Autodesk Inventor part; units mm, degrees
ref_plane "YZ Plane" through (0, 0, 0) normal (1, 0, 0) x (0, 1, 0)
ref_plane "XZ Plane" through (0, 0, 0) normal (0, 1, 0) x (-1, 0, 0)
ref_plane "XY Plane" through (0, 0, 0) normal (0, 0, 1) x (1, 0, 0)
sketch "Sketch1" plane through (0, 0, 0) normal (0, 1, 0) x (-1, 0, 0)
  circle A0 centre (0, 0) radius 1.5
  dimension "d0" = 3
extrude "Extrusion1" add sketch "Sketch1" along normal blind 10
sketch "Sketch2" plane through (0, 0, 0) normal (0, -1, 0) x (1, 0, 0)
  circle A0 centre (0, 0) radius 2.5
  dimension "d3" = 5
extrude "Extrusion2" add sketch "Sketch2" along normal blind 3
fillet "Fillet1" radius 2 1 edges at (-2.5, -3, 0)
sketch "Sketch3" plane through (0, -3, 0) normal (0, -1, 0) x (1, 0, 0)
  circle A0 centre (0, 0) radius 0.5
  line L0 (-1.8667, 0) -> (-0.4174, -0.2753)
  circle A1 centre (0, 0) radius 0.5
  line L1 (-1.8667, 0) -> (-0.5, 0)
  dimension "d9" = 0
extrude "Extrusion3" cut sketch "Sketch3" against normal blind 2 contours A0 L0 L1
mirror "Mirror1" about plane through (0, 0, 0) normal (0, 0, 1) of "Extrusion3"
pattern_circular "Circular Pattern1" count 4 over 360 about axis through (0, -1, 0) along (0, -1, 0) of "Extrusion3", "Mirror1"
sketch "Sketch4" plane through (0, -3, 0) normal (0, -1, 0) x (1, 0, 0)
  arc A0 (-0.4174, 0.2753) -> (-0.4174, -0.2753) centre (0, 0) ccw
  arc A1 (-0.4174, -0.2753) -> (-0.2753, -0.4174) centre (0, 0) ccw
  arc A2 (-0.2753, -0.4174) -> (0.2753, -0.4174) centre (0, 0) ccw
  arc A3 (0.2753, -0.4174) -> (0.4174, -0.2753) centre (0, 0) ccw
  arc A4 (0.4174, -0.2753) -> (0.4174, 0.2753) centre (0, 0) ccw
  arc A5 (0.4174, 0.2753) -> (0.2753, 0.4174) centre (0, 0) ccw
  arc A6 (0.2753, 0.4174) -> (-0.2753, 0.4174) centre (0, 0) ccw
  arc A7 (-0.2753, 0.4174) -> (-0.4174, 0.2753) centre (0, 0) ccw
extrude "Extrusion4" cut sketch "Sketch4" against normal up to surface (2 mm away)
The model under review builds one solid part; all positions refer to its coordinate system, in mm. A direction names the side the tool comes from. Round coordinates to 2 decimals unless told otherwise and drop trailing zeros. Loops run counter-clockwise (first coordinate to the right, second up) from the corner with the lowest first, then second, coordinate; pieces in that order, holes last.
Item 1: For faces 1 (the face through (0, 10, 0)), 2 (the face through (0, -1, 0)), list the 3-axis set-ups (+Z, -Z, +X, -X, +Y, -Y) from which the entire face can be reached by the end or side of a thin tool; tool diameter is ignored.
Determined:
face 1: +Z, -Z, +X, -X, +Y
face 2: -Y
Item 2: Take a section at A-A (y = 1.25). Write out the cut boundary in (x, z), then the cut area to 3 significant figures.
Determined:
outline: circle Ø3 at (0, 0)
area: 7.07 mm2
Item 3: Clearance check with flat-ended pins moving along their axes: pin 1 Ø1.5 at (x, z) = (1, 1.5) entering from -Y; pin 2 Ø1 at (x, z) = (-1.5, 1.5) entering from -Y; pin 3 Ø2 at (x, y) = (0.5, 3.5) entering from +Z. State where each tip first meets the part, or that it passes through.
Determined:
pin 1: stops at y = -2.92
pin 2: stops at y = -2.66
pin 3: stops at z = 1.5
Item 4: Mouldability with a two-part tool opening along Z and no side actions: class faces 3 (the face through (1.5, 4.93, -0.07)), 4 (the face through (-1.152, -2.014, -0.136)), 5 (the face through (1.13, -2.01, -0.14)), 6 (the face through (2, 0, 0)) as released by +Z, released by -Z, zero draft, split by the parting line, or undercut.
Determined:
face 3: split by the parting line
face 4: undercut
face 5: undercut
face 6: zero draft
Item 5: For line 1 (Y direction, x = 1.6, z = 1.05); line 2 (X direction, y = -0.5, z = -1.55); line 3 (Y direction, x = 1.2, z = 1.75), list the stretches that pass through material, from the lowest coordinate up.
Determined:
line 1: y = -2.41 to 0
line 2: x = -1.96 to 1.96
line 3: y = -2.17 to 0
